Job drawing, mm, ordinate dimensions from the low corner. One solid piece. Give positions to 0.01 mm unless a question says otherwise; leave off trailing zeros. Write each loop counter-clockwise with the first axis right and the second up, starting at its lowest first coordinate (ties: lowest second). Pieces come first, ordered by that corner, then holes. Notation, with made-up numbers: M -3,-12 L 26,-12 A34 ccw 26,27 Z; hole C 47.5,32.5 d6. An arc over 180 degrees is marked long. Use CSV: the item, a comma, the result in double quotes. Start each with the question number.
Item 1: Mould opens along X. For the marked faces 1 and 2 say: released by +X, released by -X, zero draft, split by the parting line, or undercut.
Item 2: Pin check, flat tips, straight feed: pin 1 (1.5 mm diameter, centred on y = 5.5, z = 48.5, fed in from +X); pin 2 (2.5 mm diameter, centred on y = 4, z = 25.5, fed in from +X); pin 3 (1.5 mm diameter, centred on y = 5, z = 45, fed in from -X); pin 4 (4 mm diameter, centred on x = 6.5, z = 28, fed in from -Y). Stop position of each tip, or through.
Item 3: Drill centre lines: line 1 (Z direction, x = 6.5, y = 5.25); line 2 (Z direction, x = 4.75, y = 3.5); line 3 (X direction, y = 3.75, z = 53). Where is each one in solid material? Low to high. Write a range as [from, to].
Item 4: Cut at B-B (y = 4). Count the separate pieces of the cut face and the enclosed holes in it, then the cut area to 3 significant figures.
Item 5: Cut at D-D (z = 54). List the corners of the cut face in (x, y).
Item 6: Cut at A-A (z = 25.5). List the corners of the cut face in (x, y), then the cut area to 3 significant figures.
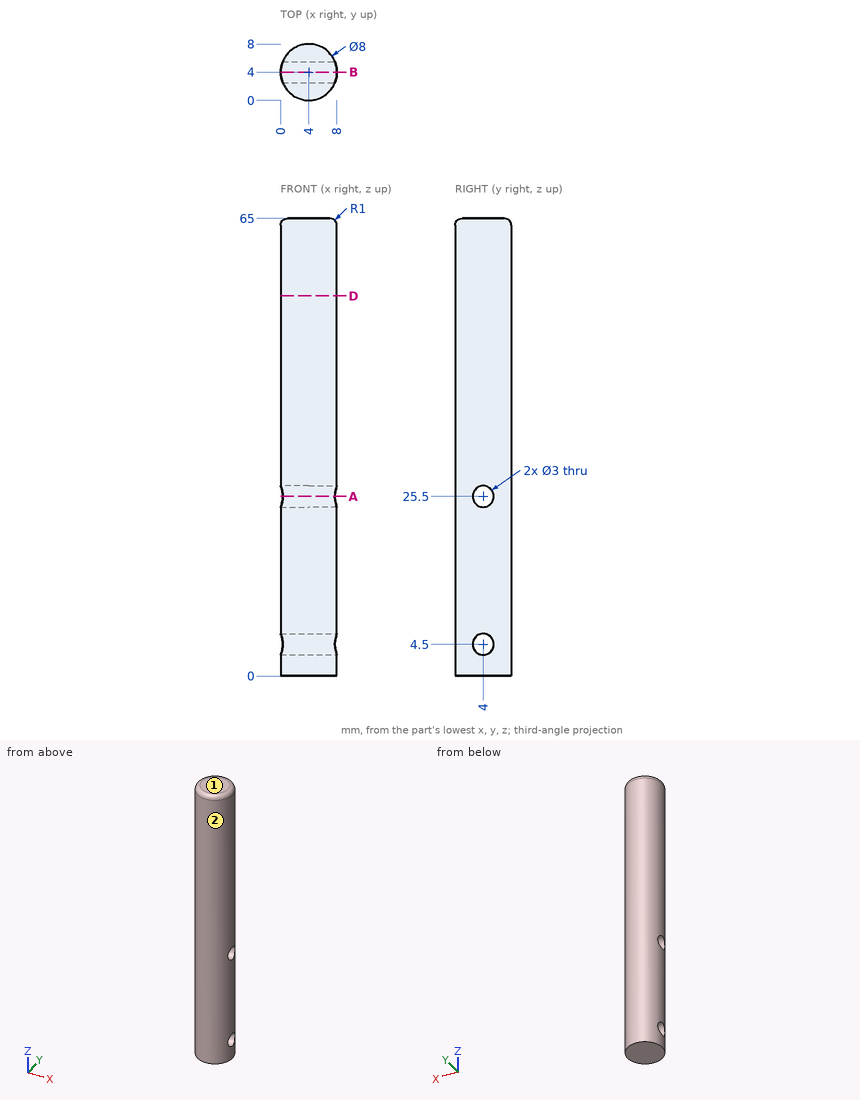
Worked answers:
1,face 1,"zero draft"
1,face 2,"split by the parting line"
2,pin 1,"stops at x = 7.93"
2,pin 2,"passes through"
2,pin 3,"stops at x = 0.01"
2,pin 4,"stops at y = 0.03"
3,line 1,"z = [0, 3.67], [5.33, 24.67], [26.33, 65]"
3,line 2,"z = [0, 3.09], [5.91, 24.09], [26.91, 65]"
3,line 3,"x = [0.01, 7.99]"
4,separate pieces,"3"
4,enclosed holes,"0"
4,area,"472 mm^2"
5,outline,"C 4,4 d8"
6,outline,"M 0.29,2.5 A4 ccw 7.71,2.5 Z; M 0.29,5.5 L 7.71,5.5 A4 ccw Z"
6,area,"26.8 mm^2"
